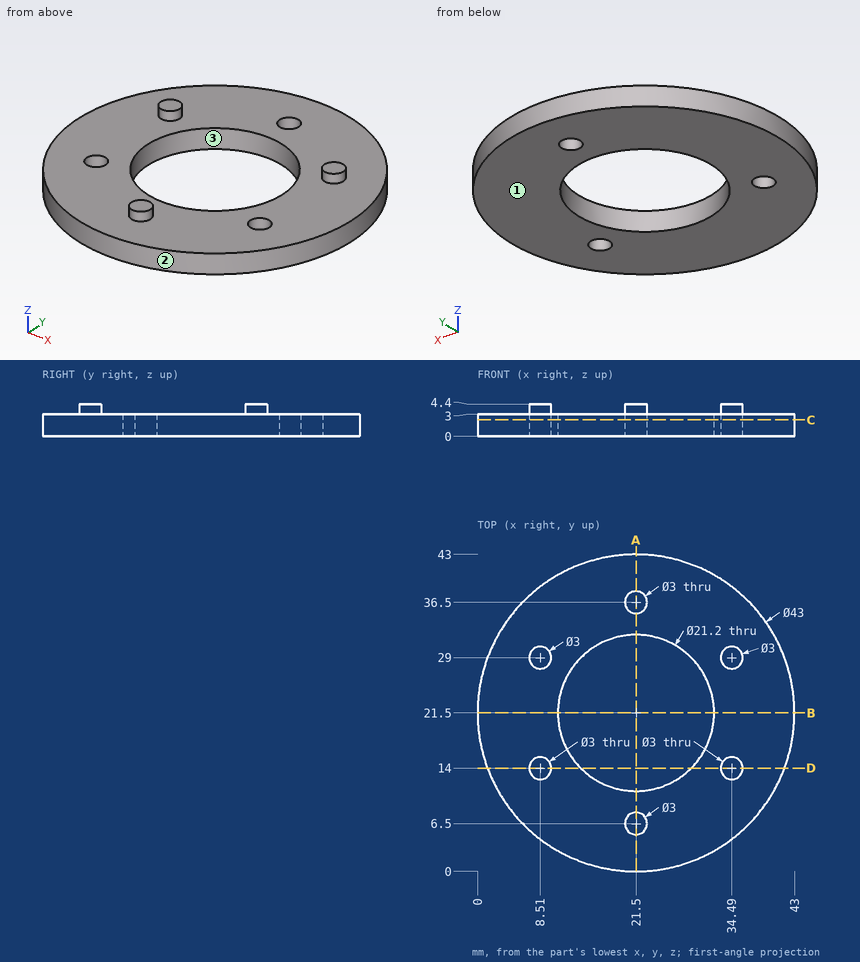
Drawing for the job (mm, zero at the part's lowest x, y, z). Round coordinates to 2 decimals unless told otherwise and drop trailing zeros. Write each loop counter-clockwise with the first axis right and the second up, starting at its lowest first coordinate (ties: lowest second). Pieces come first, ordered by that corner, then holes. Notation, with made-up numbers: (29.25, 30) - (59.25, 30) arc R23 cw to (59.25, 45) - close; hole circle Ø4 at (-1, 32). An arc over 180 degrees is marked (long way). Write item = value, one per line. Start each with the question number.
Q1. Drop flat-ended pins along their axis: pin 1 (19 mm diameter, centred on x = 21.5, y = 21.5, fed in from -Z); pin 2 (1 mm diameter, centred on y = 38, z = 2, fed in from +X); pin 3 (2 mm diameter, centred on y = 8.5, z = 1, fed in from +X); pin 4 (13 mm diameter, centred on x = 18.5, y = 15.5, fed in from +Z). Give the stop position or say it passes through.
Q2. Band-saw the part on A-A (x = 21.5). Give the cut face in (y, z), then the cut area to 3 significant figures.
Q3. Band-saw the part on C-C (z = 2.25). Give the cut face in (x, y), then the cut area to 3 significant figures.
Q4. Band-saw the part on D-D (y = 14). Give the cut face in (x, z).
Q5. Probe L1, parallel to Y at x = 21.5, z = 1.3; L2, parallel to X at y = 15, z = 1.45 (1 decimal); L3, parallel to Z at x = 25.5, y = 38. List the from-to ranges inside material, lowest first. Write a range as from..to.
Q6. Band-saw the part on B-B (y = 21.5). Give the cut face in (x, z).
Q7. Mould opens along Y. For the marked faces 1, 2 and 3 say: pulls with the +Y half, pulls with the -Y half, needs draft (parallel to the pull), parting line crosses it, or undercut.
Answers below:
q1.pin_1 = through
q1.pin_2 = 35.86
q1.pin_3 = 39.34
q1.pin_4 = 3
q2.outline = (0, 0) - (10.9, 0) - (10.9, 3) - (8, 3) - (8, 4.4) - (5, 4.4) - (5, 3) - (0, 3) - close; (32.1, 0) - (35, 0) - (35, 3) - (32.1, 3) - close; (38, 0) - (43, 0) - (43, 3) - (38, 3) - close
q2.area = 60.6 mm2
q3.outline = circle Ø43 at (21.5, 21.5); hole circle Ø3 at (8.51, 14); hole circle Ø21.2 at (21.5, 21.5); hole circle Ø3 at (21.5, 36.5); hole circle Ø3 at (34.49, 14)
q3.area = 1,080 mm2
q4.outline = (1.35, 0) - (7.01, 0) - (7.01, 3) - (1.35, 3) - close; (10.01, 0) - (14.01, 0) - (14.01, 3) - (10.01, 3) - close; (28.99, 0) - (32.99, 0) - (32.99, 3) - (28.99, 3) - close; (35.99, 0) - (41.65, 0) - (41.65, 3) - (35.99, 3) - close
q5.L1 = 0..10.9, 32.1..35, 38..43
q5.L2 = 1..7.4, 9.6..13.1, 29.9..33.4, 35.6..42
q5.L3 = 0..3
q6.outline = (0, 0) - (10.9, 0) - (10.9, 3) - (0, 3) - close; (32.1, 0) - (43, 0) - (43, 3) - (32.1, 3) - close
q7.face_1 = needs draft
q7.face_2 = parting line crosses it
q7.face_3 = undercut
